Could you check a few things on this model? Use its own coordinates, in mm. Coordinates: 2 decimals unless noted, no trailing zeros. Order: outer loops, then holes, each group sorted by start corner. A loop starts at its lowest first (then second) coordinate and runs counter-clockwise, first axis right, second up. Notation, with made-up numbers: (-17, 3.5) - (40, 3.5) arc R34 ccw to (40, 39.5) - close; hole circle Ø1 at (48, 68.5). An arc over 180 degrees is marked (long way). One line per item, written item: value. Start each with the question number.
from build123d import *

# Parameters (mm, degrees)
BOSS_EXTRUDE1_DEPTH  = 1.5875
SKETCH2_W            = 88.9
SKETCH2_H            = 203.2
SKETCH2_R            = 3.429
CUT_EXTRUDE1_DEPTH   = 2.5875
FILLET1_R            = 12.7
FILLET1_OF_MIRROR1_R = 12.7


with BuildPart() as part:
    # Sketch1 → Boss-Extrude1 (new body, symmetric)
    with BuildSketch(Plane(origin=(0, 0, 0), x_dir=(1, 0, 0), z_dir=(0, 1, 0))):
        Polygon((-314.234696616, 547.119578242), (-453.923150307, 0), (-314.234696616, -547.119578242), (0, -758.175325655), (314.234696616, -547.119578242), (453.923150307, 0), (314.234696616, 547.119578242), (0, 758.175325655), align=None)
    extrude(amount=BOSS_EXTRUDE1_DEPTH, both=True)

    # Sketch2 → Cut-Extrude1 (cut, symmetric)
    with BuildSketch(Plane(origin=(0, 0, 0), x_dir=(1, 0, 0), z_dir=(0, 1, 0))):
        with Locations((0, 381)):
            Rectangle(SKETCH2_W, SKETCH2_H)
        with Locations((-60.198, 469.9)):
            Circle(SKETCH2_R)
        with Locations((-60.198, 444.5)):
            Circle(SKETCH2_R)
        with Locations((60.198, 444.5)):
            Circle(SKETCH2_R)
        with Locations((60.198, 469.9)):
            Circle(SKETCH2_R)
    cut_extrude1 = extrude(amount=CUT_EXTRUDE1_DEPTH, both=True, mode=Mode.SUBTRACT)

    # Fillet1
    fillet1_edges = [part.edges().sort_by_distance(p)[0] for p in [
        (44.45, 0, -279.4),
        (-44.45, 0, -279.4),
        (-44.45, 0, -482.6),
        (44.45, 0, -482.6),
    ]]
    fillet(fillet1_edges, radius=FILLET1_R)

    # Mirror1: Cut-Extrude1 across plane
    add(cut_extrude1.mirror(Plane.XY), mode=Mode.SUBTRACT)

    # Fillet1 of Mirror1
    fillet1_of_mirror1_edges = [part.edges().sort_by_distance(p)[0] for p in [
        (44.45, 0, 279.4),
        (-44.45, 0, 279.4),
        (-44.45, 0, 482.6),
        (44.45, 0, 482.6),
    ]]
    fillet(fillet1_of_mirror1_edges, radius=FILLET1_OF_MIRROR1_R)


solid = part.part
Q1. I want a section at D-D on z = -172.5. Please give me the cut outline in (x, y).
Q2. If I drill on L1, parallel to X at y = -0.3, z = -469.9; L2, parallel to X at y = 0.8, z = -444.5; L3, parallel to X at y = 1.2, z = 473.5, over which ranges is the centre line in solid material (lowest first)?
Q3. I want a section at C-C on x = 381.5. Please give me the cut outline in (y, z), then the cut area to 3 significant figures.
Q4. I want a section at A-A on z = -381. Please give me the cut outline in (x, y), then the cut area to 3 significant figures.
Q5. I want a section at B-B on y = 0.5. State how many separate pieces and enclosed holes the cut face has, then the cut area to 3 significant figures.
Q6. I'm going to push flat-ended pins straight in: pin 1 (1 mm diameter, centred on y = 0.5, z = -337, fed in from -X); pin 2 (5.5 mm diameter, centred on x = 60.198, z = -469.9, fed in from -Y); pin 3 (1 mm diameter, centred on y = 1, z = 414, fed in from +X); pin 4 (1 mm diameter, centred on y = -1, z = 424, fed in from -X). Where does each tip first touch, or does it pass through?
Values follow:
1. outline: (-409.88, -1.59) - (409.88, -1.59) - (409.88, 1.59) - (-409.88, 1.59) - close
2. L1: x = -333.95 to -63.63, -56.77 to -44.45, 44.45 to 56.77, 63.63 to 333.95
2. L2: x = -340.44 to -63.63, -56.77 to -44.45, 44.45 to 56.77, 63.63 to 340.44
2. L3: x = -333.03 to -43.93, 43.93 to 333.03
3. outline: (-1.59, -283.66) - (1.59, -283.66) - (1.59, 283.66) - (-1.59, 283.66) - close
3. area: 1,800 mm^2
4. outline: (-356.65, -1.59) - (-44.45, -1.59) - (-44.45, 1.59) - (-356.65, 1.59) - close; (44.45, -1.59) - (356.65, -1.59) - (356.65, 1.59) - (44.45, 1.59) - close
4. area: 1,980 mm^2
5. separate pieces: 1
5. enclosed holes: 10
5. area: 937,000 mm^2
6. pin 1: stops at x = -368.01
6. pin 2: passes through
6. pin 3: stops at x = 348.35
6. pin 4: stops at x = -345.8
